from build123d import *

# Parameters (mm, degrees)
SKETCH1_W                      = 70
SKETCH1_H                      = 100
BOSS_EXTRUDE1_DEPTH            = 10
CBORE_FOR_M5_SHCS1_D           = 5.5
CBORE_FOR_M5_SHCS1_CBORE_D     = 10
CBORE_FOR_M5_SHCS1_CBORE_DEPTH = 5
F_1_0MM_DOWEL_HOLE1_D          = 16.3
F_1_0MM_DOWEL_HOLE1_DEPTH      = 5.3
F_1_0MM_DOWEL_HOLE3_D          = 12
SKETCH14_R                     = 3.2
CUT_EXTRUDE1_DEPTH             = 62.846584384
CHAMFER1_SIZE                  = 2


with BuildPart() as part:
    # Sketch1 → Boss-Extrude1 (new body)
    with BuildSketch(Plane(origin=(0, 0, 0), x_dir=(1, 0, 0), z_dir=(0, 1, 0))):
        Rectangle(SKETCH1_W, SKETCH1_H)
    extrude(amount=BOSS_EXTRUDE1_DEPTH)

    # CBORE for M5 SHCS1 (through all)
    with Locations(Plane(origin=(0, 10, 0), x_dir=(1, 0, 0), z_dir=(0, 1, 0))):
        with Locations((-27.5, -42.5), (-27.5, 42.5), (27.5, 42.5), (27.5, -42.5)):
            CounterBoreHole(CBORE_FOR_M5_SHCS1_D / 2, CBORE_FOR_M5_SHCS1_CBORE_D / 2, CBORE_FOR_M5_SHCS1_CBORE_DEPTH)

    # Ø1.0mm Dowel Hole1
    with Locations(Plane(origin=(0, 10, 0), x_dir=(1, 0, 0), z_dir=(0, 1, 0))):
        with Locations((0, 35)):
            Hole(F_1_0MM_DOWEL_HOLE1_D / 2, depth=F_1_0MM_DOWEL_HOLE1_DEPTH)

    # Ø1.0mm Dowel Hole3 (through all)
    with Locations(Plane(origin=(0, 4.7, 0), x_dir=(1, 0, 0), z_dir=(0, 1, 0))):
        with Locations((0, 35)):
            Hole(F_1_0MM_DOWEL_HOLE3_D / 2)

    # Sketch14 → Cut-Extrude1 (cut, through all)
    with BuildSketch(Plane(origin=(0, 10, 0), x_dir=(1, 0, 0), z_dir=(0, 1, 0))):
        with Locations(Location((12, -23.35, 0), (0, 0, 270))):
            Circle(SKETCH14_R)
        with Locations(Location((-12, -23.35, 0), (0, 0, 270))):
            Circle(SKETCH14_R)
    extrude(amount=-CUT_EXTRUDE1_DEPTH, mode=Mode.SUBTRACT)

    # Chamfer1
    chamfer1_edges = [part.edges().sort_by_distance(p)[0] for p in [
        (35, 5, 50),
        (-35, 5, 50),
        (-35, 5, -50),
        (35, 5, -50),
    ]]
    chamfer(chamfer1_edges, length=CHAMFER1_SIZE)


solid = part.part
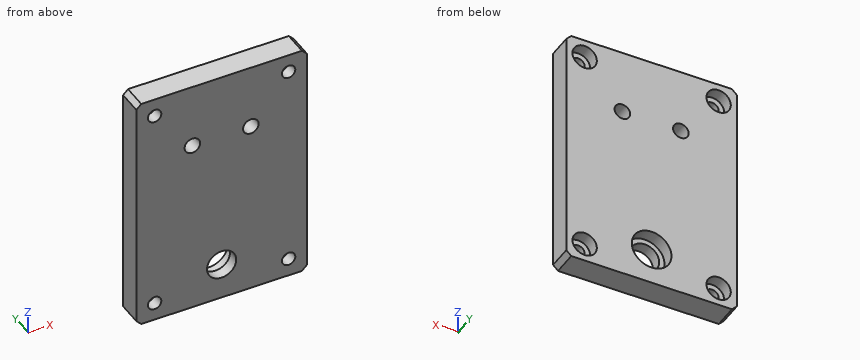
The listing builds one solid part. Answer for the finished solid, in the listing's coordinates (mm). Give positions to 0.01 mm unless a question says otherwise; leave off trailing zeros. Write each loop counter-clockwise with the first axis right and the second up, starting at its lowest first coordinate (ties: lowest second). Pieces come first, ordered by that corner, then holes.
Item 1: Find the intervals of material crossed by line 1 along Z through (x, y) = (-27.5, 1.8); line 2 along X through (y, z) = (2.8, 42.5); line 3 along X through (y, z) = (7.8, 42.5), in increasing order.
Item 2: Section D-D, the plane z = 23.35 is taken. Write down the section's boundary in (x, y), plus the area to 3 significant figures.
Item 3: Section B-B, the plane y = 1 is taken. Write down the section's boundary in (x, z), plus the area to 3 significant figures.
Item 4: Flat-ended cylindrical pins translate along their axes: P1, Ø11, axis at x = -28, z = -41.5, coming from the +Y side; P2, Ø6, axis at x = -27.5, z = -42.5, coming from the +Y side; P3, Ø6, axis at x = 12, z = 23.35, coming from the -Y side; P4, Ø15.5, axis at x = 0, z = -35, coming from the +Y side. Find the tip coordinate at first contact, or state that the pin passes through.
Item 5: Section C-C, the plane x = -12 is taken. Write down the section's boundary in (y, z).
Item 6: Section A-A, the plane z = -35 is taken. Write down the section's boundary in (x, y), plus the area to 3 significant figures.
Completed:
1. line 1: z = -50 to -45.25, -39.75 to 39.75, 45.25 to 50
1. line 2: x = -35 to -30.25, -24.75 to 24.75, 30.25 to 35
1. line 3: x = -35 to -32.5, -22.5 to 22.5, 32.5 to 35
2. outline: (-35, 0) - (-15.2, 0) - (-15.2, 10) - (-35, 10) - close; (-8.8, 0) - (8.8, 0) - (8.8, 10) - (-8.8, 10) - close; (15.2, 0) - (35, 0) - (35, 10) - (15.2, 10) - close
2. area: 572 mm2
3. outline: (-35, -48) - (-33, -50) - (33, -50) - (35, -48) - (35, 48) - (33, 50) - (-33, 50) - (-35, 48) - close; hole circle Ø5.5 at (-27.5, -42.5); hole circle Ø5.5 at (-27.5, 42.5); hole circle Ø6.4 at (-12, 23.35); hole circle Ø12 at (0, -35); hole circle Ø6.4 at (12, 23.35); hole circle Ø5.5 at (27.5, -42.5); hole circle Ø5.5 at (27.5, 42.5)
3. area: 6,720 mm2
4. P1: stops at y = 10
4. P2: stops at y = 5
4. P3: passes through
4. P4: stops at y = 4.7
5. outline: (0, -50) - (10, -50) - (10, 20.15) - (0, 20.15) - close; (0, 26.55) - (10, 26.55) - (10, 50) - (0, 50) - close
6. outline: (-35, 0) - (-6, 0) - (-6, 4.7) - (-8.15, 4.7) - (-8.15, 10) - (-35, 10) - close; (6, 0) - (35, 0) - (35, 10) - (8.15, 10) - (8.15, 4.7) - (6, 4.7) - close
6. area: 557 mm2
